from build123d import *

# Parameters (mm, degrees)
F0_W     = 2.54
F0_H     = 2.54
F1_DEPTH = 19.05
F3_DEPTH = 12.7
F4_R     = 5.08
F5_R     = 0.508
F6_R     = 0.2


with BuildPart() as f1:
    # F0 (on Right) → F1 (new body, symmetric)
    with BuildSketch(Plane.YZ):
        Polygon((-12.7, 0), (0, 0), (2.54, 0), (24.8412, 0), (24.8412, 2.54), (24.8412, 22.3012), (22.3012, 22.3012), (21.7932, 22.3012), (22.3012, 20.1749913394), (22.3012, 2.54), (2.54, 2.54), (2.54, 20.1749913394), (2.54, 22.3012), (0, 22.3012), (0, 2.54), (-10.16, 2.54), (-12.7, 2.54), align=None)
        with Locations((-11.43, 3.81)):
            Rectangle(F0_W, F0_H)
        Polygon((3.048, 22.3012), (2.54, 22.3012), (2.54, 20.1749913394), align=None)
    extrude(amount=F1_DEPTH, both=True)

    # F2 (on face) → F3 (cut, symmetric)
    with BuildSketch(Plane.XY.offset(2.54)):
        with BuildLine():
            Line((2.2225, -12.7), (2.2225, -5.08))
            ThreePointArc((2.2225, -5.08), (0, -2.8575), (-2.2225, -5.08))
            Line((-2.2225, -5.08), (-2.2225, -12.7))
            Line((-2.2225, -12.7), (2.2225, -12.7))
        make_face()
        with BuildLine():
            Line((12.85875, -12.7), (12.85875, -5.08))
            ThreePointArc((12.85875, -5.08), (10.63625, -2.8575), (8.41375, -5.08))
            Line((8.41375, -5.08), (8.41375, -12.7))
            Line((8.41375, -12.7), (12.85875, -12.7))
        make_face()
        with BuildLine():
            Line((-8.41375, -12.7), (-8.41375, -5.08))
            ThreePointArc((-8.41375, -5.08), (-10.63625, -2.8575), (-12.85875, -5.08))
            Line((-12.85875, -5.08), (-12.85875, -12.7))
            Line((-12.85875, -12.7), (-8.41375, -12.7))
        make_face()
    extrude(amount=F3_DEPTH, both=True, mode=Mode.SUBTRACT)

    # F4
    f4_edges = [f1.edges().sort_by_distance(p)[0] for p in [
        (19.05, -12.7, 2.54),
        (-19.05, -12.7, 2.54),
    ]]
    fillet(f4_edges, radius=F4_R)

    # F5
    f5_edges = [f1.edges().sort_by_distance(p)[0] for p in [
        (-18.369409, -10.16, 3.81),
        (18.369409, -10.16, 3.81),
    ]]
    fillet(f5_edges, radius=F5_R)

    # F6
    f6_edges = [f1.edges().sort_by_distance(p)[0] for p in [
        (-12.85875, -12.7, 2.54),
        (-8.41375, -12.7, 2.54),
        (-2.2225, -12.7, 2.54),
        (2.2225, -12.7, 2.54),
        (8.41375, -12.7, 2.54),
        (12.85875, -12.7, 2.54),
        (12.85875, -10.16, 3.81),
        (8.41375, -10.16, 3.81),
        (2.2225, -10.16, 3.81),
        (-2.2225, -10.16, 3.81),
        (-8.41375, -10.16, 3.81),
        (19.05, 0, 12.4206),
        (19.05, 2.54, 11.357496),
        (19.05, 2.794, 21.238096),
        (19.05, 22.3012, 11.357496),
        (19.05, 24.8412, 11.1506),
        (19.05, 22.0472, 21.238096),
        (-19.05, 0, 12.4206),
        (-19.05, 2.54, 11.357496),
        (-19.05, 22.3012, 11.357496),
        (-19.05, 24.8412, 11.1506),
        (-19.05, 22.0472, 21.238096),
        (-19.05, 2.794, 21.238096),
    ]]
    fillet(f6_edges, radius=F6_R)


solid = f1.part
The model under review builds one solid part; all positions refer to its coordinate system, in mm. A direction names the side the tool comes from. Coordinates: 2 decimals unless noted, no trailing zeros. Write each loop counter-clockwise with the first axis right and the second up, starting at its lowest first coordinate (ties: lowest second). Pieces come first, ordered by that corner, then holes. Notation, with made-up numbers: (20.25, 65) -> (75.25, 65) arc R29 ccw to (75.25, 101) -> close; hole circle Ø11 at (-24.75, 79). An arc over 180 degrees is marked (long way). Answer in a Markdown table with one row per item.
1. We need section B-B, the plane x = 0. State the section outline as (y, z) points (1 decimal).
Answers below:
| item | result |
|---|---|
| outline | (-2.9, 0) -> (24.8, 0) -> (24.8, 22.3) -> (21.8, 22.3) -> (22.3, 20.2) -> (22.3, 2.5) -> (2.5, 2.5) -> (2.5, 20.2) -> (3, 22.3) -> (0, 22.3) -> (0, 2.5) -> (-2.9, 2.5) -> close |
2. We need section C-C, the plane y = 5. State the section outline as (x, z) points.
Answers below:
| item | result |
|---|---|
| outline | (-19.05, 0) -> (19.05, 0) -> (19.05, 2.54) -> (-19.05, 2.54) -> close |
3. We need section A-A, the plane z = 19.25. State the section outline as (x, y) points.
Answers below:
| item | result |
|---|---|
| outline | (-19.05, 0.2) arc R0.2 ccw to (-18.85, 0) -> (18.85, 0) arc R0.2 ccw to (19.05, 0.2) -> (19.05, 2.34) arc R0.2 ccw to (18.85, 2.54) -> (-18.85, 2.54) arc R0.2 ccw to (-19.05, 2.34) -> close; (-19.05, 22.5) arc R0.2 ccw to (-18.85, 22.3) -> (18.85, 22.3) arc R0.2 ccw to (19.05, 22.5) -> (19.05, 24.64) arc R0.2 ccw to (18.85, 24.84) -> (-18.85, 24.84) arc R0.2 ccw to (-19.05, 24.64) -> close |
4. For faces 1 (the flat face through (-15, -11, 5.08)), 2 (the flat face through (2.222, -10, 2)), 3 (the flat face through (0, 2.54, 11)), list the 3-axis set-ups (+Z, -Z, +X, -X, +Y, -Y) from which the entire face can be reached by the end or side of a thin tool; tool diameter is ignored.
Answers below:
| item | result |
|---|---|
| face 1 | +Z, +X, -X, -Y |
| face 2 | +Z, -Z, -Y |
| face 3 | +X, -X |
5. Clearance check with flat-ended pins moving along their axes: pin 1 Ø2 at (x, y) = (15.5, -11) entering from +Z; pin 2 Ø5 at (y, z) = (-7, 6) entering from +X; pin 3 Ø4 at (y, z) = (-7.5, 3) entering from +X; pin 4 Ø5 at (x, y) = (-3, -6.5) entering from +Z. State where each tip first meets the part, or that it passes through.
Answers below:
| item | result |
|---|---|
| pin 1 | stops at z = 5.08 |
| pin 2 | passes through |
| pin 3 | stops at x = 19.05 |
| pin 4 | stops at z = 2.54 |
6. Draft analysis for pull direction Y (two halves, no side actions). For faces 4 (the flat face through (0, 24.841, 11)), 5 (the flat face through (0, 13, 2.54)), 6 (the flat face through (15, -11, 5.08)), state which applies: +Y half, -Y half, draft (parallel to the pull), parting line (faces both ways), or undercut.
Answers below:
| item | result |
|---|---|
| face 4 | +Y half |
| face 5 | undercut |
| face 6 | draft |
7. Wall thickness on probe 1 along Y at (x, z) = (8, 8.25); probe 2 along X at (y, z) = (-8.5, 2.5); probe 3 along Z at (x, y) = (-8, 14.5): over which ranges is each line inside the solid? List them lowest first. Write a range as [from, to].
Answers below:
| item | result |
|---|---|
| probe 1 | y = [0, 2.54], [22.3, 24.84] |
| probe 2 | x = [-18.97, -12.86], [-8.41, -2.22], [2.22, 8.41], [12.86, 18.97] |
| probe 3 | z = [0, 2.54] |
